Verification items for the finished model (mm, model axes). A direction names the side the tool comes from. Round coordinates to 2 decimals unless told otherwise and drop trailing zeros. Order: outer loops, then holes, each group sorted by start corner. A loop starts at its lowest first (then second) coordinate and runs counter-clockwise, first axis right, second up. Notation, with made-up numbers: (52.5, 37.25) -> (64.5, 37.25) arc R14 ccw to (64.5, 52.25) -> close; hole circle Ø1 at (2.5, 13.5). An arc over 180 degrees is marked (long way). Put each result on its own line as item: value.
```python
from build123d import *

# Parameters (mm, degrees)
SKETCH1_R           = 31.75
SKETCH1_R_2         = 25.4
BOSS_EXTRUDE3_DEPTH = 25.4
SKETCH1_3_R         = 25.4
SKETCH1_3_R_2       = 19.05
BOSS_EXTRUDE4_DEPTH = 31.75
CHAMFER1_SIZE       = 1.5875


with BuildPart() as part:
    # Sketch1 → Boss-Extrude3 (new body)
    with BuildSketch(Plane.XY):
        Circle(SKETCH1_R)
        Circle(SKETCH1_R_2, mode=Mode.SUBTRACT)
    extrude(amount=BOSS_EXTRUDE3_DEPTH)

    # Sketch1<3> → Boss-Extrude4 (add)
    with BuildSketch(Plane.XY):
        Circle(SKETCH1_3_R)
        Circle(SKETCH1_3_R_2, mode=Mode.SUBTRACT)
    extrude(amount=BOSS_EXTRUDE4_DEPTH)

    # Chamfer1
    chamfer1_edges = [part.edges().sort_by_distance(p)[0] for p in [
        (-25.4, 0, 31.75),
        (-19.05, 0, 0),
    ]]
    chamfer(chamfer1_edges, length=CHAMFER1_SIZE)


solid = part.part
```
Item 1: Material ranges on line 1 along Y through (x, z) = (0, 12); line 2 along Z through (x, y) = (-18.5, 22); line 3 along Y through (x, z) = (3.5, 29), recorded low to high.
Geometry check:
line 1: -31.75 to -19.05, 19.05 to 31.75
line 2: 0 to 25.4
line 3: -25.16 to -18.73, 18.73 to 25.16
Item 2: Tool access check on faces 4 (the face through (-11, 16, 31.75)), 5 (the face through (-14.3, 21.3, 25.4)). Record the directions out of +Z, -Z, +X, -X, +Y, -Y that give a thin tool (end or side, any length) a straight path to the whole face; none if there is none.
Geometry check:
face 4: +Z, +X, -X, +Y, -Y
face 5: +Z
Item 3: Sectioned sample at A-A, the plane x = 0. Record the boundary of the cut face in (y, z).
Geometry check:
outline: (-31.75, 0) -> (-20.64, 0) -> (-19.05, 1.59) -> (-19.05, 31.75) -> (-23.81, 31.75) -> (-25.4, 30.16) -> (-25.4, 25.4) -> (-31.75, 25.4) -> close; (19.05, 1.59) -> (20.64, 0) -> (31.75, 0) -> (31.75, 25.4) -> (25.4, 25.4) -> (25.4, 30.16) -> (23.81, 31.75) -> (19.05, 31.75) -> close
Item 4: Sectioned sample at C-C, the plane z = 3. Record the boundary of the cut face in (x, y).
Geometry check:
outline: circle Ø63.5 at (0, 0); hole circle Ø38.1 at (0, 0)
Item 5: Depth check by flat-ended pin: pin 1 Ø4 at (x, z) = (-8, 16) entering from -Y; pin 2 Ø5 at (x, z) = (21.5, 27.5) entering from +Y; pin 3 Ø1 at (x, y) = (-3, -18.5) entering from +Z; pin 4 Ø6 at (y, z) = (21.5, 9.5) entering from +X. Enter the tip coordinate at first touch or a pass-through.
Geometry check:
pin 1: y = -31.18
pin 2: y = 24.54
pin 3: z = 31.75
pin 4: x = 25.8
Item 6: Release check for a two-part mould opening along X. For faces 1 (the face through (-15.12, -11.59, 16.46)), 2 (the face through (-6.883, -30.995, 12.522)), 3 (the face through (21, 0, 0)) record: pulls with the +X half, pulls with the -X half, needs draft (parallel to the pull), parting line crosses it, or undercut.
Geometry check:
face 1: undercut
face 2: parting line crosses it
face 3: needs draft
